Input: part model. Units: mm. Frame: model coordinates. Round coordinates to 2 decimals unless told otherwise and drop trailing zeros. Loops run counter-clockwise (first coordinate to the right, second up) from the corner with the lowest first, then second, coordinate; pieces in that order, holes last. Notation, with made-up numbers: (83.25, 73.5) - (128.25, 73.5) arc R25 cw to (128.25, 103.5) - close; hole circle Ø1 at (61, -3.75). An arc over 180 degrees is marked (long way). Use CSV: the item, a comma, the result in double quotes. Start each with the question number.
1. Pin query (flat end, axial travel): P1, Ø12, axis at x = -16.29, y = 77.65, coming from the -Z side (3 decimals). Return the tip coordinate at first contact, or that it passes through.
2. Cut plane B-B (z = -1.5). Give the number of separate pieces and of enclosed holes in the cut face, and give its area (3 significant figures).
3. Pull-direction query (Y, two-part tool) for faces 1 (the cylindrical face through (-45.199, 24.516, -1.565)), 2 (the flat face through (-28.25, 85.05, -1.57)), 3 (the flat face through (-109.687, -33.159, -1.565)); classes: +Y half, -Y half, draft (parallel to the pull), parting line (faces both ways), or undercut.
4. Cut plane D-D (y = 30). Return loops of the section in (x, z) (3 decimals).
5. Cut plane C-C (x = -92.5). Return loops of the section in (y, z) (3 decimals).
6. Material intervals for probe 1 along Y at (x, z) = (-21, -2.9); probe 2 along Y at (x, z) = (-20, -0.8); probe 3 along Y at (x, z) = (-84.5, -0.6), sorted ascending. Write a range as from..to.
7. Cut plane A-A (x = -48.5). Return loops of the section in (y, z) (3 decimals).
```python
from build123d import *

# Parameters (mm, degrees)
SKETCH1_R           = 5.125
SKETCH1_R_2         = 3.175
BOSS_EXTRUDE1_DEPTH = 3.175
BOSS_EXTRUDE2_DEPTH = 3.175
FILLET1_R           = 3
FILLET2_R           = 3
SKETCH3_R           = 20
CUT_EXTRUDE1_DEPTH  = 10
FILLET3_R           = 10


with BuildPart() as part:
    # Sketch1 → Boss-Extrude1 (new body)
    with BuildSketch(Plane.XY):
        with BuildLine():
            Line((9.15916732, 81.880500013), (-1.226057593, 83.041443199))
            Line((-1.226057593, 83.041443199), (-56.039685464, 87.118947137))
            ThreePointArc((-56.039685464, 87.118947137), (-60.496641192, 86.206716079), (-63.967502721, 83.265672028))
            Line((-63.967502721, 83.265672028), (-116.255829355, 9.604754379))
            ThreePointArc((-116.255829355, 9.604754379), (-117.771483022, 6.090804864), (-117.721858217, 2.264241835))
            Line((-117.721858217, 2.264241835), (-101.423346554, -69.587878569))
            ThreePointArc((-101.423346554, -69.587878569), (-95.471980909, -76.230183562), (-86.689504727, -74.678706588))
            Line((-86.689504727, -74.678706588), (-38.949070428, -33.549176271))
            ThreePointArc((-38.949070428, -33.549176271), (-45.470819677, 24.007252392), (5.719870058, 51.114243705))
            Line((5.719870058, 51.114243705), (9.15916732, 81.880500013))
        make_face()
        with Locations((-16.285724201, 77.64676563)):
            Circle(SKETCH1_R, mode=Mode.SUBTRACT)
        with Locations((-56.48584008, 77.954801184)):
            Circle(SKETCH1_R_2, mode=Mode.SUBTRACT)
        with Locations((-108.774166869, 4.293883316)):
            Circle(SKETCH1_R_2, mode=Mode.SUBTRACT)
        with Locations((-92.47565523, -67.558236985)):
            Circle(SKETCH1_R_2, mode=Mode.SUBTRACT)
    extrude(amount=-BOSS_EXTRUDE1_DEPTH)

    # Sketch2 → Boss-Extrude2 (add)
    with BuildSketch(Plane.XY):
        with BuildLine():
            Line((9.15916732, 81.880500013), (5.719870058, 51.114243705))
            Line((5.719870058, 51.114243705), (15.657966891, 50.003284059))
            ThreePointArc((15.657966891, 50.003284059), (38.420342204, 56.582561483), (49.863520461, 77.330243105))
            Line((49.863520461, 77.330243105), (9.15916732, 81.880500013))
        make_face()
    extrude(amount=-BOSS_EXTRUDE2_DEPTH)

    # Fillet1
    fillet1_edges = [part.edges().sort_by_distance(p)[0] for p in [
        (49.863520461, 77.330243105, -1.5875),
    ]]
    fillet(fillet1_edges, radius=FILLET1_R)

    # Fillet2
    fillet2_edges = [part.edges().sort_by_distance(p)[0] for p in [
        (-38.949070428, -33.549176271, -1.5875),
    ]]
    fillet(fillet2_edges, radius=FILLET2_R)

    # Sketch3 → Cut-Extrude1 (cut)
    with BuildSketch(Plane(origin=(0, 0, -3.175), x_dir=(-1, 0, 0), z_dir=(0, 0, -1))):
        with Locations((88.139089591, 62.193219725)):
            Circle(SKETCH3_R)
    extrude(amount=-CUT_EXTRUDE1_DEPTH, mode=Mode.SUBTRACT)

    # Fillet3
    fillet3_edges = [part.edges().sort_by_distance(p)[0] for p in [
        (-71.283801873, 72.958872327, -1.5875),
        (-92.741786186, 42.730044649, -1.5875),
    ]]
    fillet(fillet3_edges, radius=FILLET3_R)


solid = part.part
```
Established:
1,P1,"stops at z = -3.175"
2,separate pieces,"1"
2,enclosed holes,"4"
2,area,"10,500 mm2"
3,face 1,"undercut"
3,face 2,"+Y half"
3,face 3,"-Y half"
4,outline,"(-101.778, -3.175) - (-41.763, -3.175) - (-41.763, 0) - (-101.778, 0) - close"
5,outline,"(-76.733, -3.175) - (-70.733, -3.175) - (-70.733, 0) - (-76.733, 0) - close; (-64.383, -3.175) - (41.103, -3.175) - (41.103, 0) - (-64.383, 0) - close"
6,probe 1,"y = 46.95..75.64, 79.66..84.51"
6,probe 2,"y = 47.38..74.12, 81.18..84.44"
6,probe 3,"y = -72.79..42.53"
7,outline,"(-41.778, -3.175) - (-17.047, -3.175) - (-17.047, 0) - (-41.778, 0) - close; (17.073, -3.175) - (86.558, -3.175) - (86.558, 0) - (17.073, 0) - close"
